Geometry check sheet. Reference: the model listing, model coordinates, mm. A direction names the side the tool comes from. Give positions to 0.01 mm unless a question says otherwise; leave off trailing zeros. Loops run counter-clockwise (first coordinate to the right, second up) from the corner with the lowest first, then second, coordinate; pieces in that order, holes last. Notation, with made-up numbers: (11.25, -40) -> (21.25, -40) arc R26 cw to (21.25, -2) -> close; hole circle Ø2 at (34.5, -31). An arc over 180 degrees is marked (long way). One line per question, with ' | ' between items.
from build123d import *

# Parameters (mm, degrees)
F1_DEPTH  = 35
F2_R      = 10
F4_DEPTH  = 35.001
F6_DEPTH  = 35.001
F7_R      = 2
F9_DEPTH  = 0.2
F10_R     = 1
F10_R_2   = 0.5
F11_DEPTH = 0.2


with BuildPart() as f1:
    # F0 (on Top) → F1 (new body)
    with BuildSketch(Plane.XY):
        Polygon((0, 110), (0, 24.7487373415), (24.7487373415, 0), (110, 0), (84.8743686708, 25.1256313292), (49.8743686708, 25.1256313292), (38.5, 13.7512626585), (27.1256313292, 25.1256313292), (25.1256313292, 25.1256313292), (25.1256313292, 27.1256313292), (13.7512626585, 38.5), (25.1256313292, 49.8743686708), (25.1256313292, 84.8743686708), align=None)
    extrude(amount=F1_DEPTH)

    # F2
    f2_edges = [f1.edges().sort_by_distance(p)[0] for p in [
        (84.874369, 25.125631, 17.5),
        (25.125631, 49.874369, 17.5),
        (25.125631, 84.874369, 17.5),
        (0, 24.748737, 17.5),
        (24.748737, 0, 17.5),
        (49.874369, 25.125631, 17.5),
    ]]
    fillet(f2_edges, radius=F2_R)

    # F3 (on face) → F4 (cut, through all)
    with BuildSketch(Plane.XY.offset(35)):
        with BuildLine():
            Line((15.1654762208, 37.0857864376), (13.7512626585, 38.5))
            Line((13.7512626585, 38.5), (13.0441558773, 37.7928932188))
            ThreePointArc((13.0441558773, 37.7928932188), (13.0441558773, 36.3786796564), (14.4583694397, 36.3786796564))
            Line((14.4583694397, 36.3786796564), (15.1654762208, 37.0857864376))
        make_face()
        with BuildLine():
            Line((37.7928932188, 13.0441558773), (38.5, 13.7512626585))
            Line((38.5, 13.7512626585), (37.0857864376, 15.1654762208))
            Line((37.0857864376, 15.1654762208), (36.3786796564, 14.4583694397))
            ThreePointArc((36.3786796564, 14.4583694397), (36.3786796564, 13.0441558773), (37.7928932188, 13.0441558773))
        make_face()
    extrude(amount=-F4_DEPTH, mode=Mode.SUBTRACT)

    # F5 (on face) → F6 (cut, through all)
    with BuildSketch(Plane.XY.offset(35)):
        with BuildLine():
            Line((8, 90.686291501), (8, 44.0624458405))
            Line((8, 44.0624458405), (16.5398448916, 52.6022907321))
            ThreePointArc((16.5398448916, 52.6022907321), (16.9733903943, 53.2511374298), (17.1256313292, 54.0165042945))
            Line((17.1256313292, 54.0165042945), (17.1256313292, 80.732233047))
            ThreePointArc((17.1256313292, 80.732233047), (16.9733903943, 81.4975999118), (16.5398448916, 82.1464466094))
            Line((16.5398448916, 82.1464466094), (8, 90.686291501))
        make_face()
        with BuildLine():
            ThreePointArc((82.1464466094, 16.5398448916), (81.4975999118, 16.9733903943), (80.732233047, 17.1256313292))
            Line((80.732233047, 17.1256313292), (54.0165042945, 17.1256313292))
            ThreePointArc((54.0165042945, 17.1256313292), (53.2511374298, 16.9733903943), (52.6022907321, 16.5398448916))
            Line((52.6022907321, 16.5398448916), (44.0624458405, 8))
            Line((44.0624458405, 8), (90.686291501, 8))
            Line((90.686291501, 8), (82.1464466094, 16.5398448916))
        make_face()
    extrude(amount=-F6_DEPTH, mode=Mode.SUBTRACT)

    # F7
    f7_edges = [f1.edges().sort_by_distance(p)[0] for p in [
        (8, 90.686292, 17.5),
        (8, 44.062446, 17.5),
        (44.062446, 8, 17.5),
        (90.686292, 8, 17.5),
    ]]
    fillet(f7_edges, radius=F7_R)

    # F8 (on face) → F9 (cut)
    with BuildSketch(Plane.XY.offset(35)):
        with BuildLine():
            ThreePointArc((18.9464101615, 24.5), (18.6, 24.7), (18.2535898385, 24.5))
            Line((18.2535898385, 24.5), (13.4038475773, 16.1))
            ThreePointArc((13.4038475773, 16.1), (13.4038475773, 15.7), (13.7502577388, 15.5))
            Line((13.7502577388, 15.5), (23.4497422612, 15.5))
            ThreePointArc((23.4497422612, 15.5), (23.7961524227, 15.7), (23.7961524227, 16.1))
            Line((23.7961524227, 16.1), (18.9464101615, 24.5))
        make_face()
        with BuildLine():
            ThreePointArc((15.9125, 18.6), (18.6, 20.075), (21.2875, 18.6))
            ThreePointArc((21.2875, 18.6), (18.6, 17.125), (15.9125, 18.6))
        make_face(mode=Mode.SUBTRACT)
    extrude(amount=-F9_DEPTH, mode=Mode.SUBTRACT)

    # F10 (on face) → F11 (cut, through all)
    with BuildSketch(Plane.XY.offset(35)):
        with Locations((18.6, 18.6)):
            Circle(F10_R)
        with Locations((18.6, 18.6)):
            Circle(F10_R_2, mode=Mode.SUBTRACT)
    extrude(amount=-F11_DEPTH, mode=Mode.SUBTRACT)


solid = f1.part
Item 1: Sectioned sample at D-D (x = 101.5). Record the cut outline in (y, z).
Result:
outline: (0, 0) -> (8.5, 0) -> (8.5, 35) -> (0, 35) -> close
Item 2: Depth check by flat-ended pin: pin 1 Ø1 at (y, z) = (26.5, 22) entering from +X; pin 2 Ø10 at (x, z) = (66.5, 26.5) entering from +Y; pin 3 Ø6 at (x, z) = (26.5, 12.5) entering from +Y. Enter the tip coordinate at first touch or a pass-through.
Result:
pin 1: x = 25.13 | pin 2: y = 25.13 | pin 3: y = 86.2
Item 3: Sectioned sample at B-B (y = 97). Record the cut outline in (x, z).
Result:
outline: (0, 0) -> (13, 0) -> (13, 35) -> (0, 35) -> close
Item 4: Release check for a two-part mould opening along Y. For faces 1 (the face through (50.075, 14.013, 17.745)), 2 (the face through (11, 99, 17)), 3 (the face through (25.013, 0.782, 17.745)), 4 (the face through (25.126, 67, 17)) record: pulls with the +Y half, pulls with the -Y half, needs draft (parallel to the pull), parting line crosses it, or undercut.
Result:
face 1: undercut | face 2: pulls with the +Y half | face 3: pulls with the -Y half | face 4: needs draft
Item 5: Sectioned sample at C-C (z = 3). Give the number of separate pieces and of enclosed holes in the cut face, plus the area to 3 significant figures.
Result:
separate pieces: 1 | enclosed holes: 2 | area: 3,020 mm2
Item 6: Set-up check for faces 5 (the face through (17.126, 67, 18)), 6 (the face through (20.215, 32.036, 17.255)), 7 (the face through (69, 0, 17)): record each of +Z, -Z, +X, -X, +Y, -Y from which the full face is reachable in a straight line by a thin tool's end or side.
Result:
face 5: +Z, -Z | face 6: +Z, -Z, +X | face 7: +Z, -Z, +X, -X, -Y
Item 7: Scan lines: probe 1 along Y at (x, z) = (68, 34.5); probe 2 along Y at (x, z) = (18.6, 34.9) (3 decimals). Record each from-to range of solid material in increasing order.
Result:
probe 1: 0 to 8, 17.13 to 25.13 | probe 2: 6.149 to 15.5, 17.125 to 17.6, 18.1 to 19.1, 19.6 to 20.075, 24.7 to 33.651, 43.349 to 91.4
Item 8: Sectioned sample at A-A (y = 59). Record the cut outline in (x, z), plus the area to 3 significant figures.
Result:
outline: (0, 0) -> (8, 0) -> (8, 35) -> (0, 35) -> close; (17.13, 0) -> (25.13, 0) -> (25.13, 35) -> (17.13, 35) -> close | area: 560 mm2
